```python
from build123d import *

# Parameters (mm, degrees)
SKETCH1_W           = 100
SKETCH1_H           = 60
BOSS_EXTRUDE1_DEPTH = 5
SKETCH2_W           = 5
SKETCH2_H           = 60
BOSS_EXTRUDE2_DEPTH = 62.3
BOSS_EXTRUDE3_DEPTH = 5
SKETCH5_R           = 35
CUT_EXTRUDE1_DEPTH  = 5


with BuildPart() as part:
    # Sketch1 → Boss-Extrude1 (new body)
    with BuildSketch(Plane(origin=(0, 0, 0), x_dir=(1, 0, 0), z_dir=(0, 1, 0))):
        with Locations((-43.057324841, 0.76433121)):
            Rectangle(SKETCH1_W, SKETCH1_H)
    extrude(amount=BOSS_EXTRUDE1_DEPTH)

    # Sketch2 → Boss-Extrude2 (add)
    with BuildSketch(Plane(origin=(0, 5, 0), x_dir=(1, 0, 0), z_dir=(0, 1, 0))):
        with Locations((4.442675159, 0.76433121)):
            Rectangle(SKETCH2_W, SKETCH2_H)
    extrude(amount=BOSS_EXTRUDE2_DEPTH)

    # Sketch4 → Boss-Extrude3 (add)
    with BuildSketch(Plane(origin=(6.942675159, 0, 0), x_dir=(0, 0, -1), z_dir=(1, 0, 0))):
        Polygon((-29.23566879, 67.3), (40.76433121, 67.3), (40.76433121, 147.3), (-39.23566879, 147.3), (-39.23566879, 67.3), align=None)
    extrude(amount=-BOSS_EXTRUDE3_DEPTH)

    # Sketch5 → Cut-Extrude1 (cut)
    with BuildSketch(Plane(origin=(6.942675159, 0, 0), x_dir=(0, 0, -1), z_dir=(1, 0, 0))):
        with Locations((0.76433121, 107.3)):
            Circle(SKETCH5_R)
    extrude(amount=-CUT_EXTRUDE1_DEPTH, mode=Mode.SUBTRACT)


solid = part.part
```
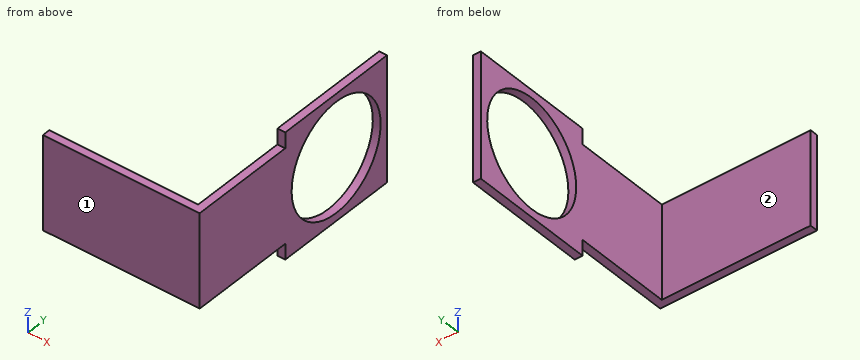
Here's how the part is built. I have some questions about the finished solid (model axes, mm). Face numbers are marked on the shaded views. A direction names the side the tool comes from. Coordinates: 2 decimals unless noted, no trailing zeros. Write each loop counter-clockwise with the first axis right and the second up, starting at its lowest first coordinate (ties: lowest second). Pieces come first, ordered by that corner, then holes. Notation, with made-up numbers: M 31.5,-32.75 L 88.5,-32.75 A9 cw 88.5,-20.75 Z; hole C 39,-9 d5. An arc over 180 degrees is marked long. Answer as CSV lines item,"result". Start each with the question number.
Q1. Suppose I cut it at A-A, the plane y = 107.3. List the corners of the cut face in (x, z) for me.
Q2. Suppose I cut it at D-D, the plane y = 127. List the corners of the cut face in (x, z) for me, then the cut area to 3 significant figures.
Q3. Suppose I cut it at C-C, the plane x = -30.5. List the corners of the cut face in (y, z) for me.
Q4. I need wall thicknesses on probe 1 along Z at (x, y) = (4, 107); probe 2 along Y at (x, z) = (-45.5, 28.5); probe 3 along X at (y, z) = (29, -26.5). Which ranges of each line are inside material? Lowest first, please. Write a range as [from, to].
Q5. Suppose I cut it at B-B, the plane z = 1.5. List the corners of the cut face in (x, y) for me, then the cut area to 3 significant figures.
Q6. For the marked faces 1 and 2, which set-ups out of +Z, -Z, +X, -X, +Y, -Y let a thin tool reach every point of the face, with its end or its side?
Q7. Will these pins go through, and if not, where does the flat tip stop? pin 1 Ø4 at (x, z) = (4.5, -37.5) entering from -Y; pin 2 Ø18 at (x, z) = (-32.5, 9) entering from +Y; pin 3 Ø1.5 at (x, z) = (-73, 19.5) entering from -Y.
Entries:
1,outline,"M 1.94,-40.76 L 6.94,-40.76 L 6.94,-35.76 L 1.94,-35.76 Z; M 1.94,34.24 L 6.94,34.24 L 6.94,39.24 L 1.94,39.24 Z"
2,outline,"M 1.94,-40.76 L 6.94,-40.76 L 6.94,-29.69 L 1.94,-29.69 Z; M 1.94,28.17 L 6.94,28.17 L 6.94,39.24 L 1.94,39.24 Z"
2,area,"111 mm²"
3,outline,"M 0,-30.76 L 5,-30.76 L 5,29.24 L 0,29.24 Z"
4,probe 1,"z = [-40.76, -35.76], [34.23, 39.24]"
4,probe 2,"y = [0, 5]"
4,probe 3,"x = [1.94, 6.94]"
5,outline,"M -93.06,0 L 6.94,0 L 6.94,72.37 L 1.94,72.37 L 1.94,5 L -93.06,5 Z; M 1.94,142.23 L 6.94,142.23 L 6.94,147.3 L 1.94,147.3 Z"
5,area,"862 mm²"
6,face 1,"+Z, -Z, +X, -X, -Y"
6,face 2,"+Z, -Z, -X, +Y"
7,pin 1,"stops at y = 67.3"
7,pin 2,"stops at y = 5"
7,pin 3,"stops at y = 0"
